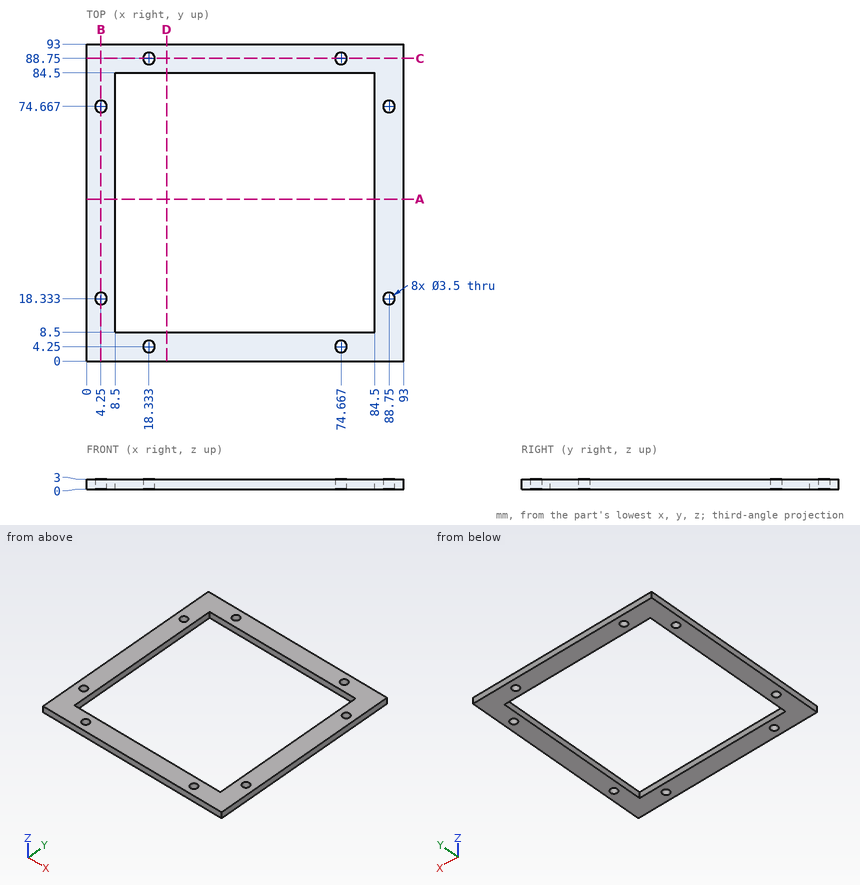
Job drawing, mm, ordinate dimensions from the low corner. One solid piece. Give positions to 0.01 mm unless a question says otherwise; leave off trailing zeros. Order: outer loops, then holes, each group sorted by start corner. A loop starts at its lowest first (then second) coordinate and runs counter-clockwise, first axis right, second up. Notation, with made-up numbers: (74.5, 22) - (83.5, 22) arc R33 ccw to (83.5, 55) - close; hole circle Ø9 at (-14.75, -34.5). An arc over 180 degrees is marked (long way). Return JSON: item names as keys, results as strings.
1) Probe line 1 (Y direction, x = 88.75, z = 1.75); line 2 (Y direction, x = 24.5, z = 1.65). List the from-to ranges inside material, lowest first. Write a range as from..to.
Geometry says:
{"line 1": "0..16.58, 20.08..72.92, 76.42..93", "line 2": "0..8.5, 84.5..93"}
2) Cut at A-A, the plane y = 47.5. Give the cut face in (x, z), plus the area to 3 significant figures.
Geometry says:
{"outline": "(0, 0) - (8.5, 0) - (8.5, 3) - (0, 3) - close; (84.5, 0) - (93, 0) - (93, 3) - (84.5, 3) - close", "area": "51.0 mm²"}
3) Cut at B-B, the plane x = 4.25. Give the cut face in (y, z), plus the area to 3 significant figures.
Geometry says:
{"outline": "(0, 0) - (16.58, 0) - (16.58, 3) - (0, 3) - close; (20.08, 0) - (72.92, 0) - (72.92, 3) - (20.08, 3) - close; (76.42, 0) - (93, 0) - (93, 3) - (76.42, 3) - close", "area": "258 mm²"}
